Model file for the job. Use its own axes, mm. Coordinates: 2 decimals unless noted, no trailing zeros. Write each loop counter-clockwise with the first axis right and the second up, starting at its lowest first coordinate (ties: lowest second). Pieces come first, ordered by that corner, then holes. Notation, with made-up numbers: (-33.75, -26.5) - (3.25, -26.5) arc R12 ccw to (3.25, -4.5) - close; hole circle Ø3 at (-32.75, 56.5). An arc over 180 degrees is marked (long way). Put each result on its own line as item: value. Start each with the question number.
1. Saw through at B-B, the plane z = 2.5. Write the cut outline in (x, y).
2. Saw through at C-C, the plane y = -23. Write the cut outline in (x, z), plus the area to 3 significant figures.
3. Drop a flat-ended pin along its axis: P1, Ø3, axis at x = -2.94, z = 2.5, coming from the -Y side. Give the stop position or say it passes through.
4. Saw through at A-A, the plane y = -2. Write the cut outline in (x, z).
5. Drill centre lines: L1, parallel to X at y = -23.25, z = 2.5; L2, parallel to X at y = 11.5, z = 2.5; L3, parallel to X at y = -8.5, z = 4.2. Where is each one in solid material? Low to high. Write a range as from..to.
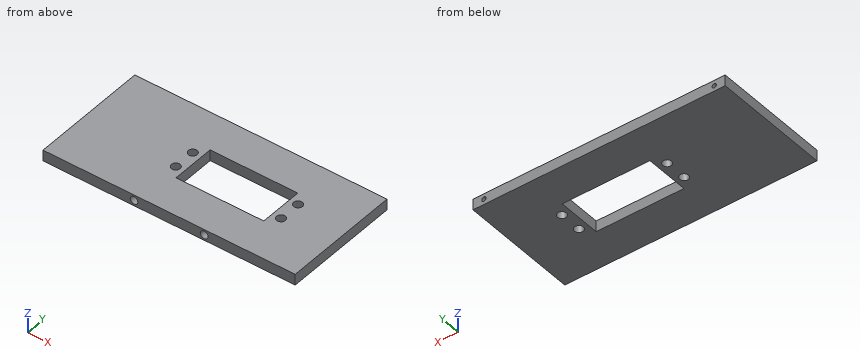
```python
from build123d import *

# Parameters (mm, degrees)
SKETCH_1_W          = 115
SKETCH_1_H          = 54
SKETCH_1_R          = 2
SKETCH_1_W_2        = 40
SKETCH_1_H_2        = 20
EXTRUDE_3_DEPTH     = 5
SKETCH_2_R          = 1
CUT_EXTRUDE_1_DEPTH = 15
SKETCH_3_R          = 1.75
CUT_EXTRUDE_2_DEPTH = 15


with BuildPart() as part:
    # 草圖1 → 填料-伸長3 (new body)
    with BuildSketch(Plane.XY):
        with Locations((13.062480584, -3.484099434)):
            Rectangle(SKETCH_1_W, SKETCH_1_H)
        with Locations((-0.937519416, -8.484099434)):
            Circle(SKETCH_1_R, mode=Mode.SUBTRACT)
        with Locations((47.062480584, -8.484099434)):
            Circle(SKETCH_1_R, mode=Mode.SUBTRACT)
        with Locations((-0.937519416, 1.515900566)):
            Circle(SKETCH_1_R, mode=Mode.SUBTRACT)
        with Locations((47.062480584, 1.515900566)):
            Circle(SKETCH_1_R, mode=Mode.SUBTRACT)
        with Locations((23.062480584, -3.484099434)):
            Rectangle(SKETCH_1_W_2, SKETCH_1_H_2, mode=Mode.SUBTRACT)
    extrude(amount=EXTRUDE_3_DEPTH)

    # 草圖2 → 除料-伸長1 (cut)
    with BuildSketch(Plane(origin=(0, 23.515900566, 0), x_dir=(1, 0, 0), z_dir=(0, 1, 0))):
        with Locations(Location((-39.437519416, -2.5, 0), (0, 0, 270))):
            Circle(SKETCH_2_R)
        with Locations(Location((65.562480584, -2.5, 0), (0, 0, 270))):
            Circle(SKETCH_2_R)
    extrude(amount=-CUT_EXTRUDE_1_DEPTH, mode=Mode.SUBTRACT)

    # 草圖3 → 除料-伸長2 (cut)
    with BuildSketch(Plane.XZ.offset(30.484099434)):
        with Locations(Location((29.062480584, 2.5, 0), (0, 0, 270))):
            Circle(SKETCH_3_R)
        with Locations(Location((-2.937519416, 2.5, 0), (0, 0, 270))):
            Circle(SKETCH_3_R)
    extrude(amount=-CUT_EXTRUDE_2_DEPTH, mode=Mode.SUBTRACT)


solid = part.part
```
Final values:
1. outline: (-44.44, -30.48) - (-4.69, -30.48) - (-4.69, -15.48) - (-1.19, -15.48) - (-1.19, -30.48) - (27.31, -30.48) - (27.31, -15.48) - (30.81, -15.48) - (30.81, -30.48) - (70.56, -30.48) - (70.56, 23.52) - (66.56, 23.52) - (66.56, 8.52) - (64.56, 8.52) - (64.56, 23.52) - (-38.44, 23.52) - (-38.44, 8.52) - (-40.44, 8.52) - (-40.44, 23.52) - (-44.44, 23.52) - close; hole circle Ø4 at (-0.94, -8.48); hole circle Ø4 at (-0.94, 1.52); hole (3.06, -13.48) - (43.06, -13.48) - (43.06, 6.52) - (3.06, 6.52) - close; hole circle Ø4 at (47.06, -8.48); hole circle Ø4 at (47.06, 1.52)
2. outline: (-44.44, 0) - (70.56, 0) - (70.56, 5) - (-44.44, 5) - close; hole circle Ø3.5 at (-2.94, 2.5); hole circle Ø3.5 at (29.06, 2.5)
2. area: 556 mm²
3. P1: stops at y = -15.48
4. outline: (-44.44, 0) - (3.06, 0) - (3.06, 5) - (-44.44, 5) - close; (43.06, 0) - (70.56, 0) - (70.56, 5) - (43.06, 5) - close
5. L1: x = -44.44..-4.69, -1.19..27.31, 30.81..70.56
5. L2: x = -44.44..-40.44, -38.44..64.56, 66.56..70.56
5. L3: x = -44.44..-2.94, 1.06..3.06, 43.06..45.06, 49.06..70.56
